```python
from build123d import *

# Parameters (mm, degrees)
BOSS_EXTRUDE1_DEPTH = 2.5
SKETCH2_R           = 1.55
BOSS_EXTRUDE2_DEPTH = 1


with BuildPart() as part:
    # Sketch1 → Boss-Extrude1 (new body)
    with BuildSketch(Plane(origin=(0, 0, 0), x_dir=(1, 0, 0), z_dir=(0, 1, 0))):
        with BuildLine():
            Line((2.5, 47.5), (2.5, 5.126263096))
            Line((2.5, 5.126263096), (5.126263096, 2.5))
            Line((5.126263096, 2.5), (47.5, 2.5))
            ThreePointArc((47.5, 2.5), (50, 0), (47.5, -2.5))
            Line((47.5, -2.5), (5.126263096, -2.5))
            Line((5.126263096, -2.5), (2.5, -5.126263096))
            Line((2.5, -5.126263096), (2.5, -47.5))
            ThreePointArc((2.5, -47.5), (0, -50), (-2.5, -47.5))
            Line((-2.5, -47.5), (-2.5, -5.126263096))
            Line((-2.5, -5.126263096), (-5.126263096, -2.5))
            Line((-5.126263096, -2.5), (-47.5, -2.5))
            ThreePointArc((-47.5, -2.5), (-50, 0), (-47.5, 2.5))
            Line((-47.5, 2.5), (-5.126263096, 2.5))
            Line((-5.126263096, 2.5), (-2.5, 5.126263096))
            Line((-2.5, 5.126263096), (-2.5, 47.5))
            ThreePointArc((-2.5, 47.5), (0, 50), (2.5, 47.5))
        make_face()
    extrude(amount=BOSS_EXTRUDE1_DEPTH)

    # Sketch2 → Boss-Extrude2 (add, symmetric)
    with BuildSketch(Plane.XY.offset(3)):
        with BuildLine():
            Line((-3, 2.5), (3, 2.5))
            Line((3, 2.5), (3, 7.5))
            ThreePointArc((3, 7.5), (0, 10.5), (-3, 7.5))
            Line((-3, 7.5), (-3, 2.5))
        make_face()
        with Locations((0, 7.5)):
            Circle(SKETCH2_R, mode=Mode.SUBTRACT)
    boss_extrude2 = extrude(amount=BOSS_EXTRUDE2_DEPTH, both=True)

    # Mirror2: Boss-Extrude2 across plane
    add(boss_extrude2.mirror(Plane.XY))


solid = part.part
```
Could you check a few things on this model? Use its own coordinates, in mm. A direction names the side the tool comes from. Give positions to 0.01 mm unless a question says otherwise; leave off trailing zeros. Loops run counter-clockwise (first coordinate to the right, second up) from the corner with the lowest first, then second, coordinate; pieces in that order, holes last. Notation, with made-up numbers: (52, -23) - (85, -23) arc R13 ccw to (85, -11) - close; hole circle Ø7 at (-38.5, 22.5). An arc over 180 degrees is marked (long way). Answer in a Markdown table with one row per item. Add a question column.
Q1. Please list where these lines run through material, in increasing order: L1, parallel to Z at x = 2, y = 3.75; L2, parallel to Y at x = 0, z = 3.2; L3, parallel to Y at x = -37, z = -1.5. Write a range as from..to.
Q2. For pin 1 (2 mm diameter, centred on y = 6, z = -3, fed in from -X); pin 2 (1.2 mm diameter, centred on y = 1.5, z = 35, fed in from +X); pin 3 (6 mm diameter, centred on x = 38, y = 4, fed in from -Z), each with a flat end and sliding along its axis, tell me the tip position at first contact or that it passes through.
Q3. Which directions (+Z, -Z, +X, -X, +Y, -Y) give clear straight access to the entire face, cutting with the end or side of a thin tool? Please do faces 1 (the face through (2.5, 1, 26)), 2 (the face through (26, 1, -2.5)), 3 (the face through (0, 5.7, 4)), 4 (the face through (-26, 1, 2.5)), 5 (the face through (-27, 1, -2.5)).
Q4. If we section it at A-A (y = 4.25): List the corners of the cut face in (x, z) for me, plus the area to 3 significant figures.
Q5. If we section it at C-C (z = -25): List the corners of the cut face in (x, y) for me, plus the area to 3 significant figures.
Q6. If we section it at B-B (x = 26.5): List the corners of the cut face in (y, z) for me.
Q7. We'd pull the mould along Z, two halves only. Please class faces 6 (the face through (27, 1, 2.5)), 7 (the face through (0.1, 10.5, -3)), 8 (the face through (50, 1, 0)), 9 (the face through (0, 5.7, -2)): +Z half, -Z half, draft (parallel to the pull), parting line (faces both ways), or undercut.
The answers:
| question | item | result |
|---|---|---|
| 1 | L1 | z = -4..-2, 2..4 |
| 1 | L2 | y = 0..5.95, 9.05..10.5 |
| 1 | L3 | y = 0..2.5 |
| 2 | pin 1 | stops at x = -3 |
| 2 | pin 2 | stops at x = 2.5 |
| 2 | pin 3 | stops at z = -2.5 |
| 3 | face 1 | +Z, +X, +Y, -Y |
| 3 | face 2 | -Z, +X, +Y, -Y |
| 3 | face 3 | +Z, +X, -X, +Y |
| 3 | face 4 | +Z, -X, +Y, -Y |
| 3 | face 5 | -Z, -X, +Y, -Y |
| 4 | outline | (-3, -4) - (3, -4) - (3, -2) - (-3, -2) - close; (-3, 2) - (3, 2) - (3, 4) - (-3, 4) - close |
| 4 | area | 24.0 mm^2 |
| 5 | outline | (-2.5, 0) - (2.5, 0) - (2.5, 2.5) - (-2.5, 2.5) - close |
| 5 | area | 12.5 mm^2 |
| 6 | outline | (0, -2.5) - (2.5, -2.5) - (2.5, 2.5) - (0, 2.5) - close |
| 7 | face 6 | +Z half |
| 7 | face 7 | draft |
| 7 | face 8 | parting line |
| 7 | face 9 | undercut |
